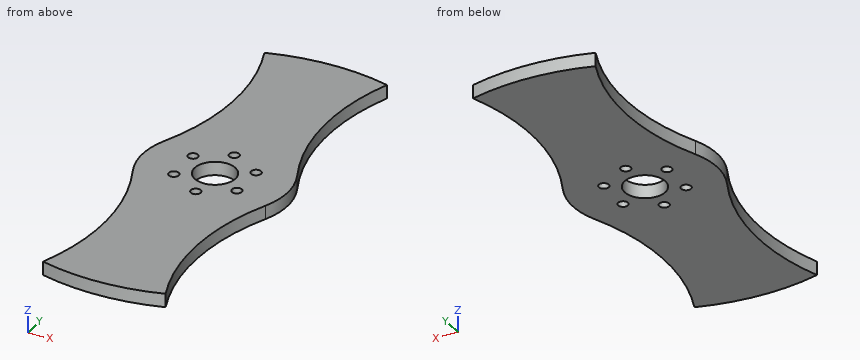
Autodesk Inventor part; units mm, degrees
ref_plane "YZ Plane" through (0, 0, 0) normal (1, 0, 0) x (0, 1, 0)
ref_plane "XZ Plane" through (0, 0, 0) normal (0, 1, 0) x (-1, 0, 0)
ref_plane "XY Plane" through (0, 0, 0) normal (0, 0, 1) x (1, 0, 0)
sketch "Sketch1" plane through (0, 0, 0) normal (0, 0, 1) x (1, 0, 0)
  circle A0 centre (0, 0) radius 7.1437
  line L0 (0, 0) -> (0, 12.7) construction
  circle A1 centre (0, 12.7) radius 1.7526
  circle A2 centre (-10.9985, 6.35) radius 1.7526
  circle A3 centre (-10.9985, -6.35) radius 1.7526
  circle A4 centre (0, -12.7) radius 1.7526
  circle A5 centre (10.9985, -6.35) radius 1.7526
  circle A6 centre (10.9985, 6.35) radius 1.7526
  circle A7 centre (0, 0) radius 76.2 construction
  line L1 (-15.875, -74.528) -> (15.875, -74.528) construction
  line L2 (15.875, -74.528) -> (15.875, 74.528) construction
  line L3 (15.875, 74.528) -> (-15.875, 74.528) construction
  line L4 (-15.875, 74.528) -> (-15.875, -74.528) construction
  line L5 (-15.875, -74.528) -> (15.875, 74.528) construction
  line L6 (15.875, -74.528) -> (-15.875, 74.528) construction
  line L7 (0, 76.2) -> (0, -76.2) construction
  line L8 (0, 0) -> (21.3699, 73.1421) construction
  circle A8 centre (0, 0) radius 66.675 construction
  circle A9 centre (0, 0) radius 25.4
  line L9 (21.3699, 73.1421) -> (17.8969, 64.2282) construction
  arc A10 (21.3699, 73.1421) -> (-21.3699, 73.1421) centre (0, 0) ccw
  line L10 (-15.875, 0) -> (15.875, 0) construction
  arc A11 (-21.3699, -73.1421) -> (21.3699, -73.1421) centre (0, 0) ccw
  arc A12 (21.3699, 73.1421) -> (23.1163, 10.5259) centre (96.4161, 43.9028) ccw
  arc A13 (-23.1163, 10.5259) -> (-21.3699, 73.1421) centre (-96.4161, 43.9028) ccw
  arc A14 (23.1163, -10.5259) -> (21.3699, -73.1421) centre (96.4161, -43.9028) ccw
  arc A15 (-21.3699, -73.1421) -> (-23.1163, -10.5259) centre (-96.4161, -43.9028) ccw
  point P0 (0, 74.528)
  point P1 (0, -66.675)
  point P2 (23.1163, -10.5259)
  point P3 (-23.1163, -10.5259)
  point P4 (-23.1163, 10.5259)
  dimension "d10" = 50.8
  dimension "d0" = 14.2875
  dimension "d1" = 12.7
  dimension "d2" = 3.5052
  dimension "d5" = 360
  dimension "d7" = 152.4
  dimension "d8" = 31.75
  dimension "d9" = 9.525
  dimension "d11" = 5
extrude "Extrusion1" add sketch "Sketch1" along normal blind 4.7625
sketch "Sketch3" plane through (0, 0, 0) normal (0, 0, -1) x (-1, 0, 0)
  circle A0 centre (0, 0) radius 76.2 construction
  point P0 (21.3699, 73.1421)
  dimension "d25" = 152.4
properties part number "Blade (Bar)" material "Stainless Steel"
Can you work these out from the model? Positions are in its coordinate system, mm. Coordinates: 2 decimals unless noted, no trailing zeros. Loops run counter-clockwise (first coordinate to the right, second up) from the corner with the lowest first, then second, coordinate; pieces in that order, holes last. Notation, with made-up numbers: (-1.75, 61.25) - (41.25, 61.25) arc R7 cw to (41.25, 71.25) - close; hole circle Ø9 at (48, 10). An arc over 180 degrees is marked (long way). Answer as a JSON object with one key per item and string values. Group by question number.
Item 1: If we section it at D-D (x = 17.5): List the corners of the cut face in (y, z) for me, plus the area to 3 significant figures.
Item 2: If we section it at C-C (z = 1.1): List the corners of the cut face in (x, y) for me.
Item 3: If we section it at A-A (x = 0): List the corners of the cut face in (y, z) for me, plus the area to 3 significant figures.
Item 4: For pin 1 (3 mm diameter, centred on x = 11, y = -6.35, fed in from -Z); pin 2 (5.5 mm diameter, centred on x = -11, y = 6.35, fed in from +Z); pin 3 (1.5 mm diameter, centred on y = 40, z = 3.5, fed in from -X); pin 4 (1 mm diameter, centred on x = -1.5, z = 3.5, fed in from +Y), each with a flat end and sliding along its axis, tell me the tip position at first contact or that it passes through.
Item 5: If I drill on L1, parallel to Y at x = 0, z = 1.4; L2, parallel to X at y = -42, z = 3; L3, parallel to X at y = -8.5, z = 1.1, over which ranges is the centre line in solid material (lowest first)? Write a range as from..to.
Item 6: If we section it at B-B (y = 0): List the corners of the cut face in (x, z) for me, plus the area to 3 significant figures.
Returned:
{
 "1": {"outline": "(-74.16, 0) - (-60, 0) - (-60, 4.76) - (-74.16, 4.76) - close; (-27.81, 0) - (27.81, 0) - (27.81, 4.76) - (-27.81, 4.76) - close; (60, 0) - (74.16, 0) - (74.16, 4.76) - (60, 4.76) - close", "area": "400 mm²"},
 "2": {"outline": "(-23.12, -10.53) arc R80.54 cw to (-21.37, -73.14) arc R76.2 ccw to (21.37, -73.14) arc R80.54 cw to (23.12, -10.53) arc R25.4 ccw to (23.12, 10.53) arc R80.54 cw to (21.37, 73.14) arc R76.2 ccw to (-21.37, 73.14) arc R80.54 cw to (-23.12, 10.53) arc R25.4 ccw to start; hole circle Ø3.51 at (-11, -6.35); hole circle Ø3.51 at (-11, 6.35); hole circle Ø14.29 at (0, 0); hole circle Ø3.51 at (0, -12.7); hole circle Ø3.51 at (0, 12.7); hole circle Ø3.51 at (11, -6.35); hole circle Ø3.51 at (11, 6.35)"},
 "3": {"outline": "(-76.2, 0) - (-14.45, 0) - (-14.45, 4.76) - (-76.2, 4.76) - close; (-10.95, 0) - (-7.14, 0) - (-7.14, 4.76) - (-10.95, 4.76) - close; (7.14, 0) - (10.95, 0) - (10.95, 4.76) - (7.14, 4.76) - close; (14.45, 0) - (76.2, 0) - (76.2, 4.76) - (14.45, 4.76) - close", "area": "624 mm²"},
 "4": {"pin 1": "passes through", "pin 2": "stops at z = 4.76", "pin 3": "stops at x = -16.01", "pin 4": "stops at y = 76.19"},
 "5": {"L1": "y = -76.2..-14.45, -10.95..-7.14, 7.14..10.95, 14.45..76.2", "L2": "x = -15.9..15.9", "L3": "x = -23.94..23.94"},
 "6": {"outline": "(-25.4, 0) - (-7.14, 0) - (-7.14, 4.76) - (-25.4, 4.76) - close; (7.14, 0) - (25.4, 0) - (25.4, 4.76) - (7.14, 4.76) - close", "area": "174 mm²"}
}
